Work out the finished part from the listing and answer in its coordinate system (mm). A direction names the side the tool comes from. Coordinates: 2 decimals unless noted, no trailing zeros. Loops run counter-clockwise (first coordinate to the right, second up) from the corner with the lowest first, then second, coordinate; pieces in that order, holes last. Notation, with made-up numbers: M -34,86.25 L -18,86.25 A7 ccw -18,90.25 Z; hole C 35.5,62.25 d7. An arc over 180 degrees is marked long. Write each question's results on one line, items separated by ' | '.
Solid Edge part; units mm, degrees
sketch "Sketch1" plane through (0, 0, 0) normal (0, -1, 0) x (1, 0, 0)
  circle A0 centre (-7.8, 73) radius 1.7
  circle A1 centre (8, 73) radius 1.7
  circle A2 centre (8, 47) radius 1.7
  circle A3 centre (-7.8, 47) radius 1.7
  line L0 (12, 79) -> (12, 41)
  line L1 (12, 41) -> (-11, 41)
  line L2 (-11, 51.3832) -> (-11, 41)
  line L3 (-11, 79) -> (-11, 68.6168)
  line L4 (12, 79) -> (-11, 79)
  arc A4 (-11, 51.3832) -> (-11, 68.6168) centre (-15, 60) ccw
extrude "Protrusion1" add sketch "Sketch1" along normal blind 9
sketch "Sketch2" plane through (-0.1, -4, 41) normal (0, 0, -1) x (-1, 0, 0)
  circle A0 centre (-0.1, 4) radius 4.2
extrude "Cutout1" cut sketch "Sketch2" against normal through all
sketch "Sketch3" plane through (-0.1, -4, 77) normal (0, 0, 1) x (-1, 0, 0)
  circle A0 centre (-0.1, -4) radius 6.2
extrude "ExtrudedCutout_2" cut sketch "Sketch3" against normal blind 1.5
sketch "Sketch4" plane through (-0.1, -4, 43) normal (0, 0, -1) x (-1, 0, 0)
  circle A0 centre (-0.1, 4) radius 6.2
extrude "ExtrudedCutout_3" cut sketch "Sketch4" against normal blind 1.5
sketch "Sketch5" plane through (12, -4.5, 61.3992) normal (1, 0, 0) x (0, 0, 1)
  line L0 (3.8779, -0.1809) -> (5.1008, -1.4472)
  line L1 (5.1008, -1.4472) -> (6.3237, -0.1809)
  arc A0 (6.3237, -0.1809) -> (3.8779, -0.1809) centre (5.1008, 1) ccw
  line L2 (-9.1221, -0.1809) -> (-7.8992, -1.4472)
  line L3 (-7.8992, -1.4472) -> (-6.6763, -0.1809)
  arc A1 (-6.6763, -0.1809) -> (-9.1221, -0.1809) centre (-7.8992, 1) ccw
extrude "Cutout2" cut sketch "Sketch5" against normal up to vertex (7 mm away)
sketch "Sketch6" plane through (-0.1, -9, 61.3992) normal (0, -1, 0) x (1, 0, 0)
  line L0 (6.9, 2.2508) -> (6.9, 7.9508)
  line L1 (6.9, 7.9508) -> (9.6, 7.9508)
  line L2 (9.6, 7.9508) -> (9.6, 2.2508)
  line L3 (9.6, 2.2508) -> (6.9, 2.2508)
  line L4 (6.9, -5.0492) -> (9.6, -5.0492)
  line L5 (9.6, -5.0492) -> (9.6, -10.7492)
  line L6 (9.6, -10.7492) -> (6.9, -10.7492)
  line L7 (6.9, -10.7492) -> (6.9, -5.0492)
extrude "Cutout3" cut sketch "Sketch6" against normal through all
sketch "Sketch7" plane through (-0.1, -9, 61.3992) normal (0, -1, 0) x (-1, 0, 0)
  circle A0 centre (-8.1, 1.3992) radius 1.7
extrude "Cutout4" cut sketch "Sketch7" against normal through all
1) Which of the six approach directions +Z, -Z, +X, -X, +Y, -Y give full straight-line access (tool end or side, diameter ignored) to faces 1 (the face through (12, -4, 60)), 2 (the face through (5.913, -3.695, 65.88)), 3 (the face through (-0.1, -6.2, 76.3)), 4 (the face through (-5, 0, 60)), 5 (the face through (8, -5, 63.65))?
Check result:
face 1: +Z, -Z, +X, +Y, -Y | face 2: +X | face 3: +Y | face 4: +Z, -Z, +X, -X, +Y | face 5: +Y, -Y
2) For a pull along X with two mould halves and no side action, classify faces 6 (the face through (5.91, -7.2, 66.56)), 7 (the face through (9.5, -4, 68)), 8 (the face through (5, -6, 66)) as released by +X, released by -X, zero draft, split by the parting line, or undercut.
Check result:
face 6: zero draft | face 7: undercut | face 8: released by +X
3) Find section A-A, the plane z = 47. Give the vertices of the cut face in (x, y), and give its area (3 significant figures).
Check result:
outline: M -11,-9 L -9.5,-9 L -9.5,0 L -11,0 Z; M -6.1,-9 L 6.3,-9 L 6.3,0 L 4.2,0 A4.2 cw -4.2,0 L -6.1,0 Z; M 9.7,-9 L 12,-9 L 12,0 L 9.7,0 Z | area: 118 mm^2
4) Find section D-D, the plane y = -1.5. Give the number of separate pieces and of enclosed holes in the cut face, and give its area (3 significant figures).
Check result:
separate pieces: 2 | enclosed holes: 7 | area: 419 mm^2
5) Find section B-B, the plane z = 60.5. Give the vertices of the cut face in (x, y), and give its area (3 significant figures).
Check result:
outline: M -5.51,-9 L 6.38,-9 L 6.38,0 L 4.2,0 A4.2 cw -4.2,0 L -5.51,0 Z; M 9.62,-9 L 12,-9 L 12,0 L 9.62,0 Z | area: 101 mm^2
6) Straight lines are drawn through the part: probe 1 along Z at (x, y) = (-3.5, -5); probe 2 along Z at (x, y) = (8, -6); probe 3 along X at (y, z) = (-4.5, 51). For each, find the intervals that lie inside material, in ascending order. Write a range as [from, to].
Check result:
probe 1: [41, 43], [44.5, 75.5], [77, 79] | probe 2: [41, 45.3], [48.7, 50.65], [56.35, 58.3], [61.7, 63.65], [69.35, 71.3], [74.7, 79] | probe 3: [-11, 6.8], [9.5, 12]
7) Given pin 1 Ø3 at (y, z) = (-3.5, 66.5) entering from -X, flat-ended and moving along its own axis, determine where the tip first touches the part or whether it passes through.
Check result:
pin 1: x = -9.88
8) Find section C-C, the plane x = 3.5. Give the vertices of the cut face in (y, z), and give its area (3 significant figures).
Check result:
outline: M -9,41 L -2.32,41 L -2.32,43 L -5.12,43 L -5.12,44.5 L -2.32,44.5 L -2.32,75.5 L -5.12,75.5 L -5.12,77 L -2.32,77 L -2.32,79 L -9,79 Z | area: 245 mm^2
